from build123d import *

# Parameters (mm, degrees)
F0_W     = 130
F0_H     = 173
F0_R     = 6.25
F0_R_2   = 17.5
F1_DEPTH = 15
F2_SIZE2 = 5
F2_SIZE  = 5


with BuildPart() as f1:
    # F0 (on Front) → F1 (new body)
    with BuildSketch(Plane.XZ):
        with Locations((5, 0)):
            Rectangle(F0_W, F0_H)
        with Locations((-41.5, -41.5)):
            Circle(F0_R, mode=Mode.SUBTRACT)
        with Locations((41.5, -41.5)):
            Circle(F0_R, mode=Mode.SUBTRACT)
        with Locations((-32.5, 0)):
            Circle(F0_R, mode=Mode.SUBTRACT)
        with Locations((-41.5, 41.5)):
            Circle(F0_R, mode=Mode.SUBTRACT)
        Circle(F0_R_2, mode=Mode.SUBTRACT)
        with Locations((32.5, 0)):
            Circle(F0_R, mode=Mode.SUBTRACT)
        with Locations((41.5, 41.5)):
            Circle(F0_R, mode=Mode.SUBTRACT)
    extrude(amount=F1_DEPTH)

    # F2
    f2_edges = [f1.edges().sort_by_distance(p)[0] for p in [
        (-47.75, -15, 41.5),
        (35.25, -15, 41.5),
        (-47.75, -15, -41.5),
        (35.25, -15, -41.5),
        (-60, -15, 0),
    ]]
    chamfer(f2_edges, length=F2_SIZE, length2=F2_SIZE2)


solid = f1.part
Design review of the part built by this model. Coordinates are the model's own, in mm. Coordinates: 2 decimals unless noted, no trailing zeros. Order: outer loops, then holes, each group sorted by start corner. A loop starts at its lowest first (then second) coordinate and runs counter-clockwise, first axis right, second up.
Item 1: For line 1 (Z direction, x = -41.5, y = -4.5); line 2 (Z direction, x = 32.5, y = -9.5); line 3 (Z direction, x = 0, y = -4), list the stretches that pass through material, from the lowest coordinate up.
Item 2: The part is to be moulded in two halves that separate along Z. For faces 1 (the flat face through (19, 0, 1)), 2 (the flat face through (4, -7, -86.5)), 3 (the conical face through (-46.71, -10.31, 37.51)), 4 (the cylindrical face through (-38.14, -4.93, -36.23)), say which applies: pulls with the +Z half, pulls with the -Z half, needs draft (parallel to the pull), parting line crosses it, or undercut.
Item 3: Take a section at C-C, the plane y = -1.75. Write out the cut boundary in (x, z).
Item 4: Take a section at A-A, the plane x = 41.5. Write out the cut boundary in (y, z).
Item 5: For pin 1 Ø14.5 at (x, z) = (-32.5, 0) entering from +Y, flat-tipped, find the tip position at first contact; note if it passes through.
Item 6: Take a section at D-D, the plane z = 0. Write out the cut boundary in (x, y).
Item 7: Take a section at B-B, the plane z = 41.5. Write out the cut boundary in (x, y).
The answers:
1. line 1: z = -86.5 to -47.75, -35.25 to 35.25, 47.75 to 86.5
1. line 2: z = -86.5 to -6.25, 6.25 to 86.5
1. line 3: z = -86.5 to -17.5, 17.5 to 86.5
2. face 1: needs draft
2. face 2: pulls with the -Z half
2. face 3: undercut
2. face 4: undercut
3. outline: (-60, -86.5) - (70, -86.5) - (70, 86.5) - (-60, 86.5) - close; hole circle Ø12.5 at (-41.5, -41.5); hole circle Ø12.5 at (-41.5, 41.5); hole circle Ø12.5 at (-32.5, 0); hole circle Ø35 at (0, 0); hole circle Ø12.5 at (32.5, 0); hole circle Ø12.5 at (41.5, -41.5); hole circle Ø12.5 at (41.5, 41.5)
4. outline: (-15, -86.5) - (0, -86.5) - (0, -47.75) - (-10, -47.75) - (-15, -52.75) - close; (-15, -30.25) - (-10, -35.25) - (0, -35.25) - (0, 35.25) - (-10, 35.25) - (-15, 30.25) - close; (-15, 52.75) - (-10, 47.75) - (0, 47.75) - (0, 86.5) - (-15, 86.5) - close
5. pin 1: stops at y = 0
6. outline: (-60, -10) - (-55, -15) - (-38.75, -15) - (-38.75, 0) - (-60, 0) - close; (-26.25, -15) - (-17.5, -15) - (-17.5, 0) - (-26.25, 0) - close; (17.5, -15) - (26.25, -15) - (26.25, 0) - (17.5, 0) - close; (38.75, -15) - (70, -15) - (70, 0) - (38.75, 0) - close
7. outline: (-60, -10) - (-55, -15) - (-52.75, -15) - (-47.75, -10) - (-47.75, 0) - (-60, 0) - close; (-35.25, -10) - (-30.25, -15) - (30.25, -15) - (35.25, -10) - (35.25, 0) - (-35.25, 0) - close; (47.75, -10) - (52.75, -15) - (70, -15) - (70, 0) - (47.75, 0) - close
